Autodesk Inventor part; units mm, degrees
ref_plane "YZ Plane" through (0, 0, 0) normal (1, 0, 0) x (0, 1, 0)
ref_plane "XZ Plane" through (0, 0, 0) normal (0, 1, 0) x (-1, 0, 0)
ref_plane "XY Plane" through (0, 0, 0) normal (0, 0, 1) x (1, 0, 0)
sketch "FrontSketch" plane through (0, 0, 0) normal (0, 0, 1) x (1, 0, 0)
  line L0 (0, 0) -> (0, 22.8261) construction
  line L1 (0, 0) -> (24.783, 0) construction
  circle A0 centre (0, 0) radius 10.25
  circle A1 centre (0, 0) radius 20.25 construction
  line L2 (-29.25, 23.25) -> (29.25, 23.25)
  line L3 (29.25, 23.25) -> (29.25, -20.25)
  line L4 (29.25, -20.25) -> (-29.25, -20.25)
  line L5 (-29.25, -20.25) -> (-29.25, 23.25)
  line L6 (0, 0) -> (-39.7334, 0) construction
  circle A2 centre (0, 0) radius 15 construction
  circle A3 centre (0, -15) radius 1.75
  line L7 (0, 0) -> (0, -25.6264) construction
  circle A4 centre (12.9904, 7.5) radius 1.75
  circle A5 centre (-12.9904, 7.5) radius 1.75
  point P0 (0, 20.25)
  point P1 (-20.25, 0)
  dimension "d25" = 30
  dimension "d21" = 20.5
  dimension "d22" = 40.5
  dimension "d23" = 9
  dimension "d24" = 3
  dimension "d26" = 3.5
  dimension "d29" = 360
extrude "Front" add sketch "FrontSketch" along normal blind 3
sketch "FerruleSketch" plane through (0, 0, 0) normal (0, 0, -1) x (-1, 0, 0)
  circle A0 centre (0, 0) radius 10.25
  line L0 (29.25, 23.25) -> (-29.25, 23.25)
  line L1 (-29.25, 23.25) -> (-29.25, -20.25)
  line L2 (-29.25, -20.25) -> (29.25, -20.25)
  line L3 (29.25, -20.25) -> (29.25, 23.25)
  circle A1 centre (0, 0) radius 20.25
  dimension "d33" = 40.5
extrude "Ferrule" add sketch "FerruleSketch" along normal blind 30 contours L3 L2 L1 L0
sketch "Sketch7" plane through (0, 0, -30) normal (0, 0, -1) x (-1, 0, 0)
  line L0 (-29.25, -20.25) -> (29.25, -20.25)
  circle A0 centre (0, 0) radius 20.25
  line L1 (-29.25, -20.25) -> (29.25, -20.25)
  line L2 (29.25, -20.25) -> (29.25, 23.25)
  line L3 (13.3229, -15.25) -> (13.3229, -20.25)
  line L4 (-13.3229, -15.25) -> (-13.3229, -20.25)
  line L5 (0, 0) -> (0, -25.3199) construction
  point P0 (0, -20.25)
  dimension "d37" = 5
extrude "Extrusion8" cut sketch "Sketch7" against normal up to surface (30 mm away) contours L4 A0 L0 | A0 L3 L0
sketch "CableHoleSketch" plane through (-29.25, 23.25, 3) normal (0, 1, 0) x (1, 0, 0)
  line L0 (0, 33) -> (58.5, 33)
  line L1 (29.25, 3) -> (29.25, 34.9321) construction
  circle A0 centre (29.25, 35) radius 4.75
  line L2 (49.5, 3) -> (9, 3)
  line L3 (24.9416, 33) -> (33.5584, 33)
  point P0 (15.9271, 3)
  point P1 (42.5729, 3)
  dimension "d40" = 32
  dimension "d41" = 9.5
extrude "CableHole" cut sketch "CableHoleSketch" against normal up to next contours L0 A0 picked at (29.25, 32.0833)
sketch "FasteningHoleSketch" plane through (-29.25, 23.25, 3) normal (0, 1, 0) x (1, 0, 0)
  arc A0 (24.9416, 33) -> (33.5584, 33) centre (29.25, 35) ccw
  line L0 (33.5584, 33) -> (58.5, 33)
  circle A1 centre (5, 5) radius 1.5
  line L1 (29.25, 3) -> (29.25, 35) construction
  line L2 (58.5, 0) -> (0, 0)
  line L3 (58.5, 0) -> (58.5, 33)
  line L4 (-10.6096, 16.5) -> (55.9901, 16.5) construction
  circle A2 centre (5, 28) radius 1.5
  line L5 (29.25, 30) -> (29.25, -2) construction
  circle A3 centre (53.5, 5) radius 1.5
  circle A4 centre (53.5, 28) radius 1.5
  dimension "d44" = 3
  dimension "d45" = 5
  dimension "d53" = 16.5
extrude "FasteningHole" cut sketch "FasteningHoleSketch" against normal blind 41.5
sketch "CoilSpringHoleSketch" plane through (-29.25, 23.25, 3) normal (0, 1, 0) x (1, 0, 0)
  circle A0 centre (53.5, 5) radius 1.5
  circle A1 centre (5, 5) radius 1.5
  circle A2 centre (5, 28) radius 1.5
  circle A3 centre (53.5, 28) radius 1.5
  arc A4 (24.9416, 33) -> (33.5584, 33) centre (29.25, 35) ccw
  line L0 (58.5, 0) -> (0, 0)
  line L1 (33.5584, 33) -> (58.5, 33)
  circle A5 centre (5, 28) radius 3
  line L2 (29.25, 3) -> (29.25, 35) construction
  line L3 (-9.4478, 16.5) -> (72.8784, 16.5) construction
  circle A6 centre (53.5, 28) radius 3
  circle A7 centre (5, 5) radius 3
  circle A8 centre (53.5, 5) radius 3
  dimension "d54" = 6
  dimension "d55" = 16.5
extrude "CoilSpringHole" cut sketch "CoilSpringHoleSketch" against normal blind 13
sketch "HollowSketch" plane through (-29.25, 23.25, 3) normal (0, 1, 0) x (1, 0, 0)
  circle A0 centre (5, 28) radius 3
  arc A1 (24.9416, 33) -> (33.5584, 33) centre (29.25, 35) ccw
  line L0 (0, 33) -> (0, 0)
  line L1 (58.5, 0) -> (0, 0)
  line L2 (0, 22.5) -> (6.75, 22.5)
  line L3 (6.75, 22.5) -> (6.75, 10.5)
  line L4 (6.75, 10.5) -> (0, 10.5)
  line L5 (0, 10.5) -> (0, 22.5)
  line L6 (29.25, 35) -> (29.25, 3) construction
  line L7 (58.5, 22.5) -> (51.75, 22.5)
  line L8 (51.75, 22.5) -> (51.75, 10.5)
  line L9 (51.75, 10.5) -> (58.5, 10.5)
  line L10 (58.5, 10.5) -> (58.5, 22.5)
  line L11 (-4.7611, 16.5) -> (67.4575, 16.5) construction
  line L12 (9.25, 35.7853) -> (9.25, -4.0496) construction
  dimension "d58" = 16.5
  dimension "d59" = 20
  dimension "d60" = 2.5
  dimension "d61" = 2.5
extrude "Hollow" cut sketch "HollowSketch" against normal up to next contours L2 L3 L4 L0 | L10 L9 L8 L7
fillet "Fillet2" radius 2 8 edges at (-22.5, 1.5, -7.5) (-29.25, 1.5, -7.5) (-22.5, 1.5, -19.5) (-29.25, 1.5, -19.5) (29.25, 1.5, -19.5) (29.25, 1.5, -7.5) (22.5, 1.5, -19.5) (22.5, 1.5, -7.5)
thread "Thread1"
thread "Thread2"
thread "Thread3"
thread "Thread4"
equation "\"d25\" = 2 * Encoder_FasteningHole_DistanceToCenter"
equation "\"d21\" = Encoder_Bearing_Diameter + EncoderSupport_PlasticShrinkingMargin"
equation "\"d22\" = Encoder_Body_Diameter + EncoderSupport_PlasticShrinkingMargin"
equation "\"d23\" = EncoderSupportInside_SideThickness"
equation "\"d24\" = EncoderSupportInside_TopThickness"
equation "\"d26\" = Encoder_FasteningHole_Diameter + EncoderSupport_PlasticShrinkingMargin"
equation "\"d33\" = Encoder_Body_Diameter + EncoderSupport_PlasticShrinkingMargin"
equation "\"d40\" = Encoder_CableBase_DistanceToTop"
equation "\"d41\" = Encoder_CableBase_Diameter + EncoderSupport_PlasticShrinkingMargin"
equation "\"d44\" = EncoderSupport_FixingHole_Diameter"
equation "\"d45\" = EncoderSupport_FixingnHole_Margin"
equation "\"d53\" = 0.5 * EncoderSupportInside_Length"
equation "\"d54\" = EncoderSupport_CoilSpringHole_Diameter"
equation "\"d55\" = 0.5 * EncoderSupportInside_Length"
equation "\"d58\" = 0.5 * EncoderSupportInside_Length"
equation "\"d59\" = 0.5 * Encoder_Body_Diameter"
equation "\"d60\" = EncoderSupportInside_Hollow_Margin"
equation "\"d61\" = EncoderSupportInside_Hollow_Margin"
equation "\"d65\" = EncoderSupport_Fillet_Size"
equation "\"EncoderSupportInside_Thickness\" = 6"
equation "\"EncoderSupportInside_Length\" = EncoderSupportInside_Front_Thickness + d34"
equation "\"EncoderSupportInside_Width\" = EncoderSupport_PlasticShrinkingMargin + Encoder_Body_Diameter + 2 * EncoderSupportInside_SideThickness"
equation "\"EncoderSupportInside_Height\" = EncoderSupport_PlasticShrinkingMargin + Encoder_Body_Diameter + EncoderSupportInside_Thickness"
equation "\"EncoderSupport_FixingHole_Diameter\" = 3"
equation "\"EncoderSupport_FixingnHole_Margin\" = 5"
equation "\"EncoderSupportInside_SideThickness\" = EncoderSupportInside_Thickness + EncoderSupport_FixingHole_Diameter"
equation "\"EncoderSupport_CoilSpringHole_Diameter\" = 6"
equation "\"EncoderSupportInside_TopThickness\" = 3"
equation "\"EncoderSupportInside_Hollow_Margin\" = 2.5"
equation "\"EncoderSupport_Fillet_Size\" = 2"
equation "\"EncoderSupport_PlasticShrinkingMargin\" = 0.5"
properties part number "EncoderSupportInside" material "Polyethylene, High Density"
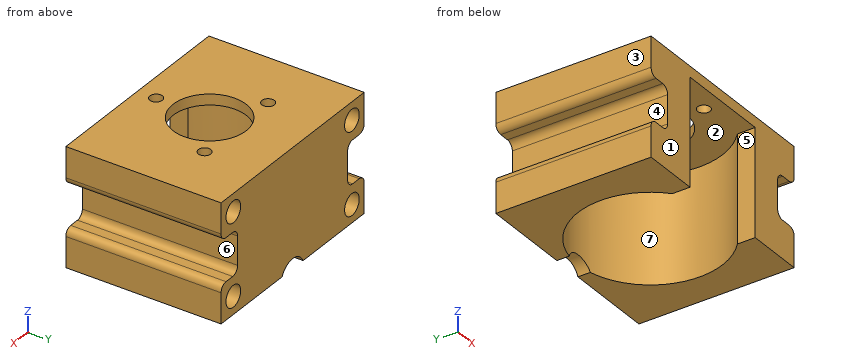
Verification items for the finished model (mm, model axes). Face numbers are marked on the shaded views. A direction names the side the tool comes from. Coordinates: 2 decimals unless noted, no trailing zeros. Order: outer loops, then holes, each group sorted by start corner. A loop starts at its lowest first (then second) coordinate and runs counter-clockwise, first axis right, second up. Notation, with made-up numbers: M 79,31.5 L 128,31.5 A8 cw 128,40.5 Z; hole C 69.25,-13 d5. An arc over 180 degrees is marked long. One line per item, written item: value. Start each with the question number.
Item 1: Sectioned sample at A-A (y = 0). Count the separate pieces of the cut face and the enclosed holes in it, then the cut area to 3 significant figures.
Item 2: Gauge pin test, flat ends, axial feed: pin 1 (3 mm diameter, centred on x = -9, y = 8.5, fed in from -Z); pin 2 (0.9 mm diameter, centred on x = 24.5, z = -2, fed in from +Y); pin 3 (4 mm diameter, centred on y = 9, z = -14.5, fed in from -X). Record the tip position at first contact, or that the pin passes through.
Item 3: Sectioned sample at B-B (z = -25). Enter the section's corners in (x, y), then the cut area to 3 significant figures.
Item 4: Sectioned sample at C-C (y = 11). Enter the section's corners in (x, z), then the cut area to 3 significant figures.
Item 5: Mould release check, pull along Y, two halves, no side actions. Record for the marked faces 1, 2 and 3: released by +Y, released by -Y, zero draft, split by the parting line, or undercut.
Item 6: Sectioned sample at D-D (x = 16.5). Enter the section's corners in (y, z).
Item 7: Access from +Z, -Z, +X, -X, +Y, -Y to the whole of each face (thin tool, end or side, straight path). Record for the marked faces 4, 5, 6 and 7.
Item 8: Scan lines: probe 1 along Z at (x, y) = (-24.25, 13.75); probe 2 along X at (y, z) = (4.5, -3); probe 3 along X at (y, z) = (-13, -3). Record each from-to range of solid material in increasing order.
Conclusion:
1. separate pieces: 2
1. enclosed holes: 4
1. area: 464 mm^2
2. pin 1: stops at z = 0
2. pin 2: stops at y = -18.25
2. pin 3: stops at x = -22.5
3. outline: M -29.25,-20.25 L -13.32,-20.25 L -13.32,-15.25 A20.25 cw long 13.32,-15.25 L 13.32,-20.25 L 29.25,-20.25 L 29.25,23.25 L 27.25,23.25 L 27.25,10.25 L 25.75,10.25 L 25.75,-18.25 L 22.75,-18.25 L 22.75,10.25 L 21.25,10.25 L 21.25,23.25 L -21.25,23.25 L -21.25,10.25 L -22.75,10.25 L -22.75,-18.25 L -25.75,-18.25 L -25.75,10.25 L -27.25,10.25 L -27.25,23.25 L -29.25,23.25 Z
3. area: 888 mm^2
4. outline: M -29.25,-30 L -17,-30 L -17,0 L 17,0 L 17,-30 L 29.25,-30 L 29.25,-21.5 A2 ccw 27.25,-19.5 L 24.5,-19.5 A2 cw 22.5,-17.5 L 22.5,-9.5 A2 cw 24.5,-7.5 L 27.25,-7.5 A2 ccw 29.25,-5.5 L 29.25,3 L -29.25,3 L -29.25,-5.5 A2 ccw -27.25,-7.5 L -24.5,-7.5 A2 cw -22.5,-9.5 L -22.5,-17.5 A2 cw -24.5,-19.5 L -27.25,-19.5 A2 ccw -29.25,-21.5 Z; hole C -24.25,-25 d6; hole C -24.25,-2 d6; hole C 24.25,-25 d6; hole C 24.25,-2 d6
4. area: 635 mm^2
5. face 1: released by -Y
5. face 2: undercut
5. face 3: zero draft
6. outline: M -20.25,-30 L -11.74,-30 L -11.74,0 L 11.74,0 L 11.74,-30 L 23.25,-30 L 23.25,3 L -20.25,3 Z
7. face 4: -X, +Y, -Y
7. face 5: -Z, -Y
7. face 6: +X, +Y, -Y
7. face 7: -Z
8. probe 1: z = -30 to -28, -22 to -19.48, -7.52 to -5, 1 to 3
8. probe 2: x = -29.25 to -25.37, -23.13 to -19.74, 19.74 to 23.13, 25.37 to 29.25
8. probe 3: x = -29.25 to -25.37, -23.13 to -15.53, 15.53 to 23.13, 25.37 to 29.25
